Here's the drawing with two shaded views (mm, measured from the low corner). I have some questions. A direction names the side the tool comes from. Coordinates: 2 decimals unless noted, no trailing zeros. Write each loop counter-clockwise with the first axis right and the second up, starting at its lowest first coordinate (ties: lowest second). Pieces come first, ordered by that corner, then holes.
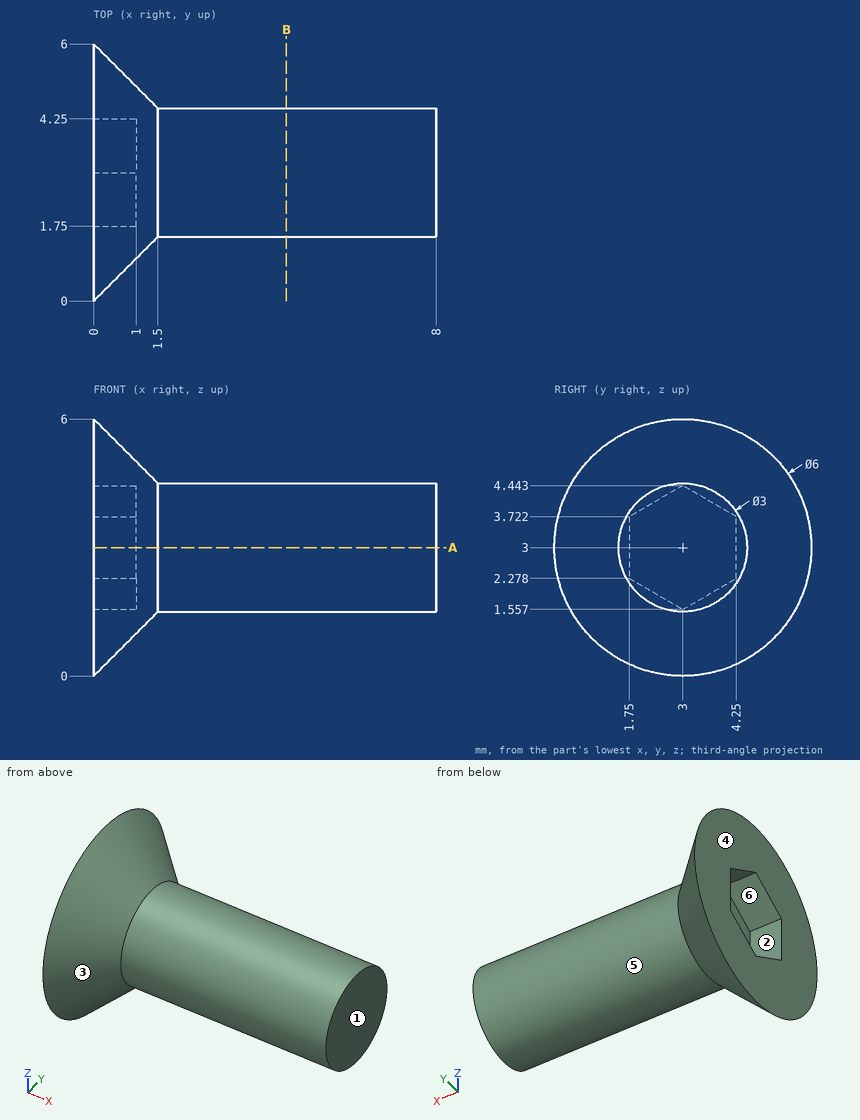
1. If I drill on L1, parallel to X at y = 4.05, z = 3.4; L2, parallel to Y at x = 3, z = 3.4 (1 decimal); L3, parallel to X at y = 2.35, z = 5.65, over which ranges is the centre line in solid material (lowest first)?
2. Which directions (+Z, -Z, +X, -X, +Y, -Y) give clear straight access to the entire face, cutting with the end or side of a thin tool? Please do the marked faces 4, 5 and 6.
3. If we section it at B-B, the plane x = 4.5: List the corners of the cut face in (y, z) for me.
4. We'd pull the mould along Z, two halves only. Please class the marked faces 1, 2 and 3: released by +Z, released by -Z, zero draft, split by the parting line, or undercut.
5. If we section it at A-A, the plane z = 3: List the corners of the cut face in (x, y) for me.
6. I'm going to push flat-ended pins straight in: P1, Ø1, axis at x = 7, z = 3, coming from the -Y side; P2, Ø3, axis at x = 3.5, y = 4.5, coming from the +Z side; P3, Ø0.5, axis at x = 0.5, z = 2.5, coming from the -Y side. Where does each tip first touch, or does it pass through?
Answers:
1. L1: x = 1 to 8
1. L2: y = 1.6 to 4.4
1. L3: x = 0 to 0.27
2. face 4: +Z, -Z, -X, +Y, -Y
2. face 5: +X
2. face 6: -X
3. outline: circle Ø3 at (3, 3)
4. face 1: zero draft
4. face 2: undercut
4. face 3: split by the parting line
5. outline: (0, 0) - (1.5, 1.5) - (8, 1.5) - (8, 4.5) - (1.5, 4.5) - (0, 6) - (0, 4.25) - (1, 4.25) - (1, 1.75) - (0, 1.75) - close
6. P1: stops at y = 1.5
6. P2: stops at z = 4.5
6. P3: stops at y = 0.29
